from build123d import *

# Parameters (mm, degrees)
SKETCH1_W                                           = 81.999999998
SKETCH1_H                                           = 60
BOSS_EXTRUDE1_DEPTH                                 = 19
TAP_DRILL_FOR_M6_TAP1_D                             = 5
CSK_FOR_M6_COUNTERSUNK_FLAT_HEAD_SCREW1_D           = 6.6
CSK_FOR_M6_COUNTERSUNK_FLAT_HEAD_SCREW1_CSINK_D     = 12.6
CSK_FOR_M6_COUNTERSUNK_FLAT_HEAD_SCREW1_CSINK_ANGLE = 90
SKETCH7_W                                           = 81.999999998
SKETCH7_H                                           = 14.054377775
BOSS_EXTRUDE2_DEPTH                                 = 19
TAP_DRILL_FOR_M5_TAP1_D                             = 4.2
TAP_DRILL_FOR_M5_TAP1_DEPTH                         = 30
TAP_DRILL_FOR_M5_TAP1_TIP                           = 1.2618073
FILLET1_R                                           = 4


with BuildPart() as part:
    # Sketch1 → Boss-Extrude1 (new body)
    with BuildSketch(Plane.XY):
        with Locations((20.999999999, 42.839007865)):
            Rectangle(SKETCH1_W, SKETCH1_H)
    extrude(amount=BOSS_EXTRUDE1_DEPTH)

    # Tap Drill for M6 Tap1 (through all)
    with Locations(Plane.XY.offset(19)):
        with Locations((8.999999998, 62.839007865), (54.999999998, 62.839007865)):
            Hole(TAP_DRILL_FOR_M6_TAP1_D / 2)

    # CSK for M6 Countersunk Flat Head Screw1 (through all)
    with Locations(Plane.XY.offset(19)):
        with Locations((0, 19.839007865), (0, 49.839007865)):
            CounterSinkHole(CSK_FOR_M6_COUNTERSUNK_FLAT_HEAD_SCREW1_D / 2, CSK_FOR_M6_COUNTERSUNK_FLAT_HEAD_SCREW1_CSINK_D / 2, counter_sink_angle=CSK_FOR_M6_COUNTERSUNK_FLAT_HEAD_SCREW1_CSINK_ANGLE)

    # Sketch7 → Boss-Extrude2 (add)
    with BuildSketch(Plane.XY.offset(19)):
        with Locations((20.999999999, 5.816196753)):
            Rectangle(SKETCH7_W, SKETCH7_H)
    extrude(amount=-BOSS_EXTRUDE2_DEPTH)

    # Tap Drill for M5 Tap1
    with Locations(Plane(origin=(0, -1.210992135, 0), x_dir=(-1, 0, 0), z_dir=(0, -1, 0))):
        with Locations((-41.999999998, -9.5)):
            Hole(TAP_DRILL_FOR_M5_TAP1_D / 2, depth=TAP_DRILL_FOR_M5_TAP1_DEPTH)
            with Locations((0, 0, -(TAP_DRILL_FOR_M5_TAP1_DEPTH + TAP_DRILL_FOR_M5_TAP1_TIP / 2))):  # 118° drill point
                Cone(0, TAP_DRILL_FOR_M5_TAP1_D / 2, TAP_DRILL_FOR_M5_TAP1_TIP, mode=Mode.SUBTRACT)

    # Fillet1
    fillet1_edges = [part.edges().sort_by_distance(p)[0] for p in [
        (-20, -1.210992135, 9.5),
        (61.999999998, -1.210992135, 9.5),
        (-20, 72.839007865, 9.5),
        (61.999999998, 72.839007865, 9.5),
    ]]
    fillet(fillet1_edges, radius=FILLET1_R)


solid = part.part
The model under review builds one solid part; all positions refer to its coordinate system, in mm. Give positions to 0.01 mm unless a question says otherwise; leave off trailing zeros. Write each loop counter-clockwise with the first axis right and the second up, starting at its lowest first coordinate (ties: lowest second). Pieces come first, ordered by that corner, then holes.
1. Wall thickness on L1, parallel to Y at x = 0, z = 8.5; L2, parallel to X at y = 18, z = 9.5; L3, parallel to Y at x = 55, z = 8.75: over which ranges is each line inside the solid? List them lowest first.
2. For P1, Ø1.5, axis at x = 45.5, y = 52, coming from the -Z side, flat-tipped, find the tip position at first contact; note if it passes through.
3. Add section A-A, the plane x = 0. Write out the cut boundary in (y, z), plus the area to 3 significant figures.
4. Add section B-B, the plane x = 9. Write out the cut boundary in (y, z), plus the area to 3 significant figures.
5. Draft analysis for pull direction Y (two halves, no side actions). For faces 1 (the cylindrical face through (-18.86, -0.01, 9.37)), 2 (the conical face through (0.747, 16.475, 16.146)), 3 (the cylindrical face through (43.13, 14, 7.73)), 4 (the flat face through (20, 72.839, 9)), state which applies: +Y half, -Y half, draft (parallel to the pull), parting line (faces both ways), or undercut.
Worked answers:
1. L1: y = -1.21 to 16.54, 23.14 to 46.54, 53.14 to 72.84
1. L2: x = -20 to -2.74, 2.74 to 39.9, 44.1 to 62
1. L3: y = -1.21 to 60.34, 65.34 to 72.84
2. P1: stops at z = 0
3. outline: (-1.21, 0) - (16.54, 0) - (16.54, 16) - (13.54, 19) - (-1.21, 19) - close; (23.14, 0) - (46.54, 0) - (46.54, 16) - (43.54, 19) - (26.14, 19) - (23.14, 16) - close; (53.14, 0) - (72.84, 0) - (72.84, 19) - (56.14, 19) - (53.14, 16) - close
3. area: 1,140 mm2
4. outline: (-1.21, 0) - (60.34, 0) - (60.34, 19) - (-1.21, 19) - close; (65.34, 0) - (72.84, 0) - (72.84, 19) - (65.34, 19) - close
4. area: 1,310 mm2
5. face 1: -Y half
5. face 2: undercut
5. face 3: draft
5. face 4: +Y half
